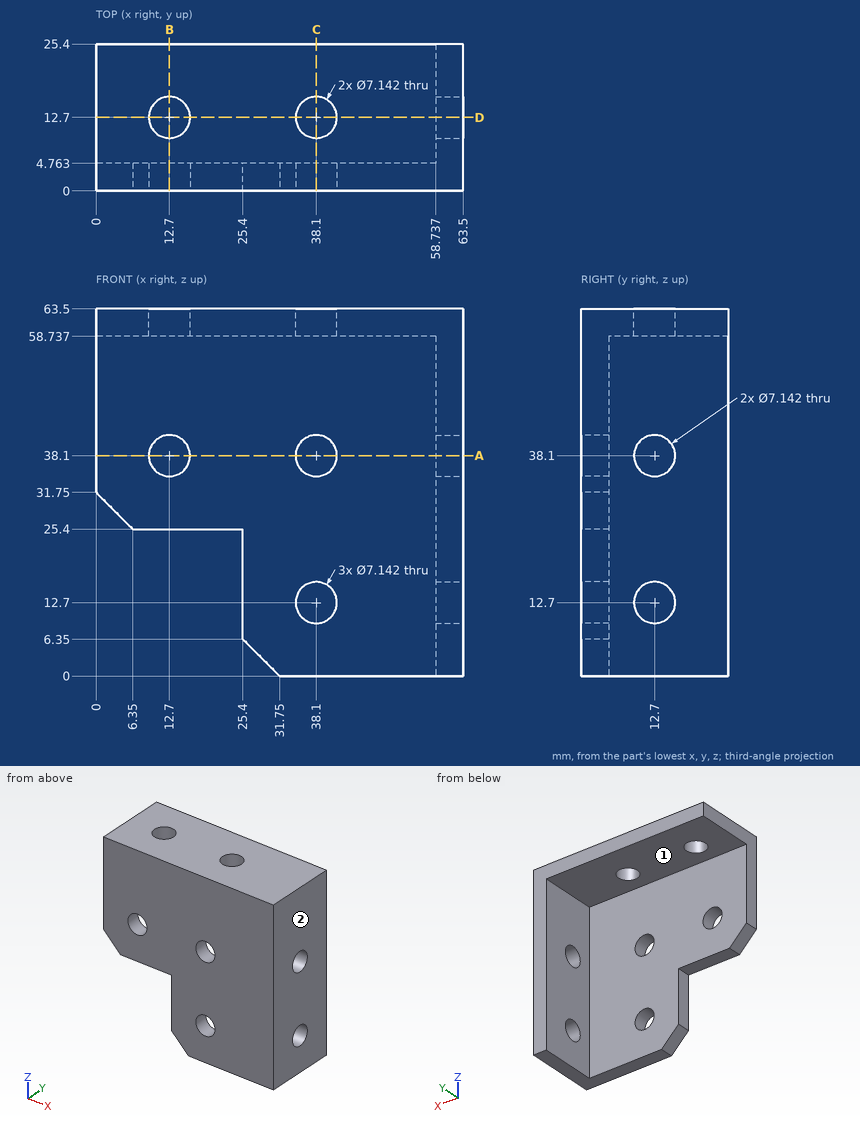
Could you check a few things on this drawing? It's one solid part, dimensions in mm from its lowest x, y, z. A direction names the side the tool comes from. Coordinates: 2 decimals unless noted, no trailing zeros. Order: outer loops, then holes, each group sorted by start corner. A loop starts at its lowest first (then second) coordinate and runs counter-clockwise, first axis right, second up. Notation, with made-up numbers: (58, 18) - (101, 18) arc R26 cw to (101, 49) - close; hole circle Ø10 at (-2.75, 34.5). An arc over 180 degrees is marked (long way). One line per question, with ' | ' between items. Start each with the question number.
1. If we section it at D-D (y = 12.7): Write out the boundary of the cut face in (x, z), and give its area (3 significant figures).
2. Which directions (+Z, -Z, +X, -X, +Y, -Y) give clear straight access to the entire face, cutting with the end or side of a thin tool? Please do the marked faces 1 and 2.
3. If we section it at A-A (z = 38.1): Write out the boundary of the cut face in (x, y).
4. If we section it at C-C (x = 38.1): Write out the boundary of the cut face in (y, z).
5. If we section it at B-B (x = 12.7): Write out the boundary of the cut face in (y, z).
6. Please list where these lines run through material, in increasing order: line 1 along Y through (x, z) = (59.95, 12.7); line 2 along Z through (x, y) = (37, 4.5); line 3 along Z through (x, y) = (32.5, 21.75). Write a range as [from, to].
7. I'm going to push flat-ended pins straight in: pin 1 Ø6 at (y, z) = (19.5, 25.5) entering from -X; pin 2 Ø6 at (x, y) = (13, 22.5) entering from -Z; pin 3 Ø5 at (y, z) = (3, 16.5) entering from -X. Where does each tip first touch, or does it pass through?
Model answer:
1) outline: (0, 58.74) - (9.13, 58.74) - (9.13, 63.5) - (0, 63.5) - close; (16.27, 58.74) - (34.53, 58.74) - (34.53, 63.5) - (16.27, 63.5) - close; (41.67, 58.74) - (58.74, 58.74) - (58.74, 41.67) - (63.5, 41.67) - (63.5, 63.5) - (41.67, 63.5) - close; (58.74, 0) - (63.5, 0) - (63.5, 9.13) - (58.74, 9.13) - close; (58.74, 16.27) - (63.5, 16.27) - (63.5, 34.53) - (58.74, 34.53) - close | area: 446 mm²
2) face 1: -Z, -X, +Y | face 2: +Z, -Z, +X, +Y, -Y
3) outline: (0, 0) - (9.13, 0) - (9.13, 4.76) - (0, 4.76) - close; (16.27, 0) - (34.53, 0) - (34.53, 4.76) - (16.27, 4.76) - close; (41.67, 0) - (63.5, 0) - (63.5, 9.13) - (58.74, 9.13) - (58.74, 4.76) - (41.67, 4.76) - close; (58.74, 16.27) - (63.5, 16.27) - (63.5, 25.4) - (58.74, 25.4) - close
4) outline: (0, 0) - (4.76, 0) - (4.76, 9.13) - (0, 9.13) - close; (0, 16.27) - (4.76, 16.27) - (4.76, 34.53) - (0, 34.53) - close; (0, 41.67) - (4.76, 41.67) - (4.76, 58.74) - (9.13, 58.74) - (9.13, 63.5) - (0, 63.5) - close; (16.27, 58.74) - (25.4, 58.74) - (25.4, 63.5) - (16.27, 63.5) - close
5) outline: (0, 25.4) - (4.76, 25.4) - (4.76, 34.53) - (0, 34.53) - close; (0, 41.67) - (4.76, 41.67) - (4.76, 58.74) - (9.13, 58.74) - (9.13, 63.5) - (0, 63.5) - close; (16.27, 58.74) - (25.4, 58.74) - (25.4, 63.5) - (16.27, 63.5) - close
6) line 1: y = [0, 9.13], [16.27, 25.4] | line 2: z = [0, 9.3], [16.1, 34.7], [41.5, 63.5] | line 3: z = [58.74, 63.5]
7) pin 1: stops at x = 58.74 | pin 2: stops at z = 58.74 | pin 3: stops at x = 25.4
